Read the model definition and answer for the solid it produces. Units are mm, in the model's axes. Face numbers are marked on the shaded views. A direction names the side the tool comes from. Give positions to 0.01 mm unless a question says otherwise; leave off trailing zeros. Order: outer loops, then holes, each group sorted by start corner. A loop starts at its lowest first (then second) coordinate and runs counter-clockwise, first axis right, second up. Notation, with made-up numbers: (-13, 23.25) -> (17, 23.25) arc R26 cw to (17, 38.25) -> close; hole circle Ø5 at (-38.75, 6.25). An arc over 180 degrees is marked (long way). Answer as CSV lines item,"result". Start each with the question number.
1) The mould has two halves that part along X. Classify the marked faces 6, 7 and 8: +X half, -X half, draft (parallel to the pull), parting line (faces both ways), or undercut.
2) Find section A-A (z = 5.5). Determine the outline of the cut face in (x, y), and give its area (3 significant figures).
3) Find section D-D (z = 11). State how many separate pieces and enclosed holes the cut face has, and give its area (3 significant figures).
4) Find section C-C (y = 9.5). Determine the outline of the cut face in (x, z), and give its area (3 significant figures).
5) For the marked faces 1, 2, 3, 4 and 5, determine the directions among +Z, -Z, +X, -X, +Y, -Y from which every point of the face is accessible in a straight line to the end or side of a thin tool.
6) Find section B-B (z = -8.5). Determine the outline of the cut face in (x, y).
7) Flat-ended cylindrical pins translate along their axes: pin 1 Ø6 at (y, z) = (32.5, 4) entering from -X; pin 2 Ø4 at (y, z) = (18.37, 11) entering from +X; pin 3 Ø0.5 at (y, z) = (3.5, -5) entering from -X. Find the tip coordinate at first contact, or state that the pin passes through.
8) Straight lines are drawn through the part: L1, parallel to X at y = 3.35, z = 11; L2, parallel to X at y = 3.6, z = -6; L3, parallel to X at y = 37, z = 8.75. For each, find the intervals that lie inside material, in ascending order. Write a range as from..to.
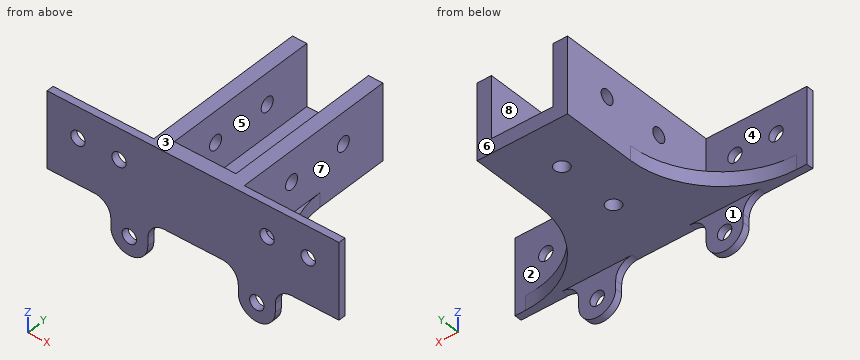
```python
from build123d import *

# Parameters (mm, degrees)
SKETCH1_W           = 22
SKETCH1_H           = 42
BOSS_EXTRUDE1_DEPTH = 18.5
SKETCH2_W           = 15
SKETCH2_H           = 38.5
CUT_EXTRUDE1_DEPTH  = 15
SKETCH3_W           = 24.5
SKETCH3_H           = 1.75
BOSS_EXTRUDE2_DEPTH = 18.5
BOSS_EXTRUDE3_DEPTH = 3.5
SKETCH5_R           = 1.75
BOSS_EXTRUDE4_DEPTH = 1.75
SKETCH6_R           = 1.75
CUT_EXTRUDE2_DEPTH  = 10
FILLET1_R           = 4
SKETCH7_R           = 1.75
CUT_EXTRUDE3_DEPTH  = 28
SKETCH8_R           = 1.75
CUT_EXTRUDE4_DEPTH  = 28


with BuildPart() as part:
    # Sketch1 → Boss-Extrude1 (new body)
    with BuildSketch(Plane.XY):
        with Locations((-5.139289452, 23.868914656)):
            Rectangle(SKETCH1_W, SKETCH1_H)
    extrude(amount=BOSS_EXTRUDE1_DEPTH)

    # Sketch2 → Cut-Extrude1 (cut)
    with BuildSketch(Plane.XY.offset(18.5)):
        with Locations((-5.139289452, 25.618914656)):
            Rectangle(SKETCH2_W, SKETCH2_H)
    extrude(amount=-CUT_EXTRUDE1_DEPTH, mode=Mode.SUBTRACT)

    # Sketch3 → Boss-Extrude2 (add)
    with BuildSketch(Plane(origin=(0, 0, 0), x_dir=(-1, 0, 0), z_dir=(0, 0, -1))):
        with Locations((28.389289452, 3.743914656)):
            Rectangle(SKETCH3_W, SKETCH3_H)
        with Locations((-18.110710548, 3.743914656)):
            Rectangle(SKETCH3_W, SKETCH3_H)
    extrude(amount=-BOSS_EXTRUDE2_DEPTH)

    # Sketch4 → Boss-Extrude3 (add)
    with BuildSketch(Plane(origin=(0, 0, 0), x_dir=(-1, 0, 0), z_dir=(0, 0, -1))):
        with BuildLine():
            Line((38.139289452, 4.618914656), (16.139289452, 4.618914656))
            Line((16.139289452, 4.618914656), (16.139289452, 26.618914656))
            ThreePointArc((16.139289452, 26.618914656), (22.582940266, 11.06256547), (38.139289452, 4.618914656))
        make_face()
        with BuildLine():
            Line((-27.860710548, 4.618914656), (-5.860710548, 4.618914656))
            Line((-5.860710548, 4.618914656), (-5.860710548, 26.618914656))
            ThreePointArc((-5.860710548, 26.618914656), (-12.304361361, 11.06256547), (-27.860710548, 4.618914656))
        make_face()
    extrude(amount=-BOSS_EXTRUDE3_DEPTH)

    # Sketch5 → Boss-Extrude4 (add)
    # profile 1 of 2: a face of its own
    with BuildSketch(Plane.XZ.offset(-2.868914656)):
        with BuildLine():
            Line((14.860710548, -6), (14.860710548, 0))
            Line((14.860710548, 0), (5.860710548, 0))
            Line((5.860710548, 0), (5.860710548, -6))
            ThreePointArc((5.860710548, -6), (10.360710548, -10.5), (14.860710548, -6))
        make_face()
        with Locations(Location((10.360710548, -6, 0), (0, 0, 270))):
            Circle(SKETCH5_R, mode=Mode.SUBTRACT)
    # profile 2 of 2: a face of its own
    with BuildSketch(Plane.XZ.offset(-2.868914656)):
        with BuildLine():
            Line((-25.139289452, -6), (-25.139289452, 0))
            Line((-25.139289452, 0), (-16.139289452, 0))
            Line((-16.139289452, 0), (-16.139289452, -6))
            ThreePointArc((-16.139289452, -6), (-20.639289452, -10.5), (-25.139289452, -6))
        make_face()
        with Locations(Location((-20.639289452, -6, 0), (0, 0, 270))):
            Circle(SKETCH5_R, mode=Mode.SUBTRACT)
    extrude(amount=-BOSS_EXTRUDE4_DEPTH)

    # Sketch6 → Cut-Extrude2 (cut)
    with BuildSketch(Plane(origin=(0, 4.618914656, 0), x_dir=(1, 0, 0), z_dir=(0, 1, 0))):
        with Locations(Location((22.860710548, -11, 0), (0, 0, 270))):
            Circle(SKETCH6_R)
        with Locations(Location((-33.139289452, -11, 0), (0, 0, 270))):
            Circle(SKETCH6_R)
        with Locations(Location((12.860710548, -11, 0), (0, 0, 270))):
            Circle(SKETCH6_R)
        with Locations(Location((-23.139289452, -11, 0), (0, 0, 270))):
            Circle(SKETCH6_R)
    extrude(amount=-CUT_EXTRUDE2_DEPTH, mode=Mode.SUBTRACT)

    # Fillet1
    fillet1_edges = [part.edges().sort_by_distance(p)[0] for p in [
        (14.860710548, 3.743914656, 0),
        (5.860710548, 3.743914656, 0),
        (-25.139289452, 3.743914656, 0),
        (-16.139289452, 3.743914656, 0),
    ]]
    fillet(fillet1_edges, radius=FILLET1_R)

    # Sketch7 → Cut-Extrude3 (cut)
    with BuildSketch(Plane.ZY.offset(16.139289452)):
        with Locations(Location((11, 33.368914656, 0), (0, 0, 270))):
            Circle(SKETCH7_R)
        with Locations(Location((11, 18.368914656, 0), (0, 0, 270))):
            Circle(SKETCH7_R)
    extrude(amount=-CUT_EXTRUDE3_DEPTH, mode=Mode.SUBTRACT)

    # Sketch8 → Cut-Extrude4 (cut)
    with BuildSketch(Plane(origin=(0, 0, 0), x_dir=(-1, 0, 0), z_dir=(0, 0, -1))):
        with Locations((5.139289452, 33.368914656)):
            Circle(SKETCH8_R)
        with Locations((5.139289452, 18.368914656)):
            Circle(SKETCH8_R)
    extrude(amount=-CUT_EXTRUDE4_DEPTH, mode=Mode.SUBTRACT)


solid = part.part
```
Findings below:
1,face 6,"draft"
1,face 7,"+X half"
1,face 8,"undercut"
2,outline,"(-40.64, 2.87) -> (30.36, 2.87) -> (30.36, 4.62) -> (5.86, 4.62) -> (5.86, 44.87) -> (2.36, 44.87) -> (2.36, 6.37) -> (-12.64, 6.37) -> (-12.64, 44.87) -> (-16.14, 44.87) -> (-16.14, 4.62) -> (-40.64, 4.62) -> close"
2,area,"432 mm²"
3,separate pieces,"9"
3,enclosed holes,"0"
3,area,"359 mm²"
4,outline,"(-24.32, 0) -> (14.04, 0) -> (14.04, 3.5) -> (5.86, 3.5) -> (5.86, 18.5) -> (2.36, 18.5) -> (2.36, 3.5) -> (-12.64, 3.5) -> (-12.64, 18.5) -> (-16.14, 18.5) -> (-16.14, 3.5) -> (-24.32, 3.5) -> close"
4,area,"239 mm²"
5,face 1,"-Z, +X, -X, +Y"
5,face 2,"+Z, +X, +Y"
5,face 3,"+Z, +X, -X, +Y, -Y"
5,face 4,"+Z, -X, +Y"
5,face 5,"+Z, +Y"
6,outline,"(-24.38, 2.87) -> (-16.9, 2.87) -> (-16.9, 4.62) -> (-24.38, 4.62) -> close; (6.62, 2.87) -> (14.1, 2.87) -> (14.1, 4.62) -> (6.62, 4.62) -> close"
7,pin 1,"x = -16.14"
7,pin 2,"x = 5.86"
7,pin 3,"x = -25.14"
8,L1,"-40.64..-34.89, -31.39..-24.89, -21.39..11.11, 14.61..21.11, 24.61..30.36"
8,L2,"-25.14..-22.39, -18.89..-16.14, 5.86..8.61, 12.11..14.86"
8,L3,"-16.14..-12.64, 2.36..5.86"
